Read the model definition and answer for the solid it produces. Units are mm, in the model's axes. Face numbers are marked on the shaded views. A direction names the side the tool comes from. Coordinates: 2 decimals unless noted, no trailing zeros. Order: outer loops, then holes, each group sorted by start corner. A loop starts at its lowest first (then second) coordinate and runs counter-clockwise, first axis right, second up. Notation, with made-up numbers: M -35,46.25 L 15,46.25 A29 ccw 15,67.25 Z; hole C 84.25,72.5 d7. An arc over 180 degrees is marked long. One line per question, with ' | ' between items. Start each with the question number.
1) Find section D-D, the plane z = 3. Write down the section's boundary in (x, y).
2) Given P1, Ø6.5, axis at y = 11, z = -2.5, coming from the +X side; P2, Ø5, axis at x = 20.5, z = 0, coming from the -Y side; P3, Ø1, axis at x = 39, y = -19, coming from the -Z side; P4, Ø2.5, axis at x = 0.5, z = -4.5, coming from the -Y side, each flat-ended and moving along its own axis, determine where each tip first touches the part or whether it passes through.
3) Find section C-C, the plane z = -4. Count the separate pieces of the cut face and the enclosed holes in it, plus the area to 3 significant figures.
4) Consider probe 1 along X at (y, z) = (33, -2.5); probe 2 along X at (y, z) = (-8.5, -5.25); probe 3 along Y at (x, z) = (3.5, -1). Determine where each line is inside the solid, lowest interval first.
5) The mould has two halves that part along X. Classify the marked faces 1 and 2: +X half, -X half, draft (parallel to the pull), parting line (faces both ways), or undercut.
6) Find section A-A, the plane y = 0. Write down the section's boundary in (x, z), plus the area to 3 significant figures.
7) Find section B-B, the plane x = 0. Write down the section's boundary in (y, z).
8) A tool of negligible diameter and unlimited length cuts with its end or side. For the marked faces 3 and 4, from which of +Z, -Z, +X, -X, +Y, -Y can it reach the whole face along a straight path? Write none if from no direction.
from build123d import *

# Parameters (mm, degrees)
SKETCH1_R           = 50
BOSS_EXTRUDE1_DEPTH = 5
SKETCH2_W           = 34
SKETCH2_H           = 70
BOSS_EXTRUDE3_DEPTH = 8
SKETCH3_W           = 27
SKETCH3_H           = 63
CUT_EXTRUDE1_DEPTH  = 8
SKETCH4_W           = 4
SKETCH4_H           = 4
CUT_EXTRUDE2_DEPTH  = 99.939375377
LPATTERN1_COUNT     = 3
LPATTERN1_PITCH     = 10
SKETCH5_W           = 4
SKETCH5_H           = 4
CUT_EXTRUDE3_DEPTH  = 84.982140959
LPATTERN2_COUNT     = 8
LPATTERN2_PITCH     = 8


with BuildPart() as part:
    # Sketch1 → Boss-Extrude1 (new body)
    with BuildSketch(Plane.XY):
        Circle(SKETCH1_R)
    extrude(amount=BOSS_EXTRUDE1_DEPTH)

    # Sketch2 → Boss-Extrude3 (add)
    with BuildSketch(Plane(origin=(0, 0, 0), x_dir=(-1, 0, 0), z_dir=(0, 0, -1))):
        Rectangle(SKETCH2_W, SKETCH2_H)
    extrude(amount=BOSS_EXTRUDE3_DEPTH)

    # Sketch3 → Cut-Extrude1 (cut)
    with BuildSketch(Plane(origin=(0, 0, -8), x_dir=(-1, 0, 0), z_dir=(0, 0, -1))):
        Rectangle(SKETCH3_W, SKETCH3_H)
    extrude(amount=-CUT_EXTRUDE1_DEPTH, mode=Mode.SUBTRACT)

    # Sketch4 → Cut-Extrude2 (cut, through all)
    with BuildSketch(Plane.XZ.offset(35)):
        with Locations((-10, -4)):
            Rectangle(SKETCH4_W, SKETCH4_H)
    cut_extrude2 = extrude(amount=-CUT_EXTRUDE2_DEPTH, mode=Mode.SUBTRACT)

    # LPattern1: Cut-Extrude2 ×3
    with Locations(*[(i * LPATTERN1_PITCH, 0, 0) for i in range(1, LPATTERN1_COUNT)]):
        add(cut_extrude2, mode=Mode.SUBTRACT)

    # Sketch5 → Cut-Extrude3 (cut, through all)
    with BuildSketch(Plane.ZY.offset(17)):
        with Locations((-4, 28)):
            Rectangle(SKETCH5_W, SKETCH5_H)
    cut_extrude3 = extrude(amount=-CUT_EXTRUDE3_DEPTH, mode=Mode.SUBTRACT)

    # LPattern2: Cut-Extrude3 ×8
    with Locations(*[(0, -i * LPATTERN2_PITCH, 0) for i in range(1, LPATTERN2_COUNT)]):
        add(cut_extrude3, mode=Mode.SUBTRACT)


solid = part.part
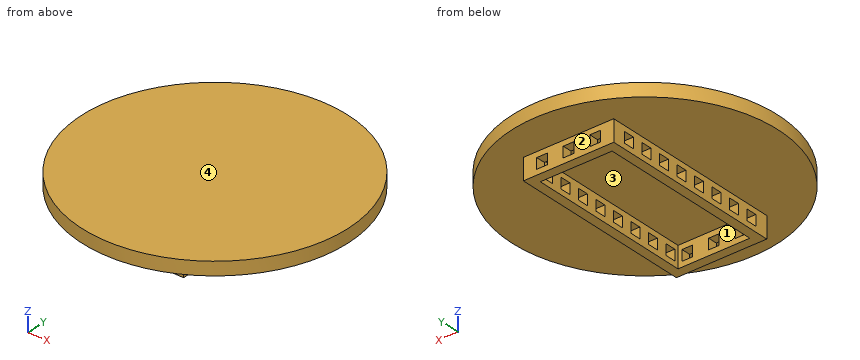
Report:
1) outline: C 0,0 d100
2) P1: stops at x = 49.2 | P2: stops at y = -46.65 | P3: stops at z = 0 | P4: passes through
3) separate pieces: 22 | enclosed holes: 0 | area: 371 mm^2
4) probe 1: x = -17 to -12, -8 to -2, 2 to 8, 12 to 17 | probe 2: x = -17 to -13.5, 13.5 to 17 | probe 3: y = -35 to -31.5, 31.5 to 35
5) face 1: undercut | face 2: draft
6) outline: M -50,0 L -17,0 L -17,-8 L -13.5,-8 L -13.5,0 L 13.5,0 L 13.5,-8 L 17,-8 L 17,0 L 50,0 L 50,5 L -50,5 Z | area: 556 mm^2
7) outline: M -50,0 L -35,0 L -35,-2 L -31.5,-2 L -31.5,0 L 31.5,0 L 31.5,-2 L 35,-2 L 35,0 L 50,0 L 50,5 L -50,5 Z; M -35,-8 L -31.5,-8 L -31.5,-6 L -35,-6 Z; M 31.5,-8 L 35,-8 L 35,-6 L 31.5,-6 Z
8) face 3: -Z | face 4: +Z, +X, -X, +Y, -Y
